Can you work these out from the model? Positions are in its coordinate system, mm. A direction names the side the tool comes from. Coordinates: 2 decimals unless noted, no trailing zeros. Order: outer loops, then holes, each group sorted by start corner. A loop starts at its lowest first (then second) coordinate and runs counter-clockwise, first axis right, second up. Notation, with made-up numbers: (5.5, 87.25) -> (40.5, 87.25) arc R38 ccw to (40.5, 125.25) -> close; hole circle Ø5 at (5, 67.25). An arc over 180 degrees is marked (long way). Answer in a Markdown table with one row per item. Add a question column.
1. Imagine slicing it at C-C on y = 82.5. Write out the boundary of the cut face in (x, z).
2. We'd pull the mould along Y, two halves only. Please class faces 3 (the face through (-2, 29, 25)), 4 (the face through (71, -82, 13)), 5 (the face through (-2, -122.5, 12)): pulls with the +Y half, pulls with the -Y half, needs draft (parallel to the pull), parting line crosses it, or undercut.
3. Will these pins go through, and if not, where does the flat tip stop? pin 1 (15.5 mm diameter, centred on x = 120, y = 82.5, fed in from -Z); pin 2 (8.5 mm diameter, centred on x = 124, y = 82.5, fed in from +Z).
4. Imagine slicing it at B-B on y = 0. Write out the boundary of the cut face in (x, z), plus the area to 3 significant figures.
5. Imagine slicing it at D-D on x = 65. Write out the boundary of the cut face in (y, z).
6. On a 3-axis mill with a long thin cutter (end or side, diameter ignored), from which of +Z, -Z, +X, -X, +Y, -Y can I reach the whole of each face in a straight line? I mean faces 1 (the face through (-114, 83, 13)), 2 (the face through (-2, 122.5, 12)). Say none if no direction works.
7. Imagine slicing it at A-A on x = 0. Write out the boundary of the cut face in (y, z), plus the area to 4 significant figures.
8. If I drill on line 1 along X through (y, z) = (82.5, 4.75); line 2 along X through (y, z) = (-82.5, 7.5); line 3 along Y through (x, z) = (-65, 4.75), over which ranges is the centre line in solid material (lowest first)? Write a range as [from, to].
from build123d import *

# Parameters (mm, degrees)
SKETCH1_W           = 280
SKETCH1_H           = 245
SKETCH1_R           = 5.25
SKETCH1_R_2         = 6
BOSS_EXTRUDE1_DEPTH = 25
SKETCH2_R           = 8.5
CUT_EXTRUDE1_DEPTH  = 12


with BuildPart() as part:
    # Sketch1 → Boss-Extrude1 (new body)
    with BuildSketch(Plane.XY):
        Rectangle(SKETCH1_W, SKETCH1_H)
        with Locations((-120, 82.5)):
            Circle(SKETCH1_R, mode=Mode.SUBTRACT)
        with Locations((120, 82.5)):
            Circle(SKETCH1_R, mode=Mode.SUBTRACT)
        with Locations((-65, -82.5)):
            Circle(SKETCH1_R, mode=Mode.SUBTRACT)
        with Locations((65, -82.5)):
            Circle(SKETCH1_R, mode=Mode.SUBTRACT)
        Circle(SKETCH1_R_2, mode=Mode.SUBTRACT)
    extrude(amount=BOSS_EXTRUDE1_DEPTH)

    # Sketch2 → Cut-Extrude1 (cut)
    with BuildSketch(Plane.XY.offset(25)):
        with Locations((-120, 82.5)):
            Circle(SKETCH2_R)
        with Locations((120, 82.5)):
            Circle(SKETCH2_R)
        with Locations((65, -82.5)):
            Circle(SKETCH2_R)
        with Locations((-65, -82.5)):
            Circle(SKETCH2_R)
    extrude(amount=-CUT_EXTRUDE1_DEPTH, mode=Mode.SUBTRACT)


solid = part.part
Answers follow:
| question | item | result |
|---|---|---|
| 1 | outline | (-140, 0) -> (-125.25, 0) -> (-125.25, 13) -> (-128.5, 13) -> (-128.5, 25) -> (-140, 25) -> close; (-114.75, 0) -> (114.75, 0) -> (114.75, 13) -> (111.5, 13) -> (111.5, 25) -> (-111.5, 25) -> (-111.5, 13) -> (-114.75, 13) -> close; (125.25, 0) -> (140, 0) -> (140, 25) -> (128.5, 25) -> (128.5, 13) -> (125.25, 13) -> close |
| 2 | face 3 | needs draft |
| 2 | face 4 | undercut |
| 2 | face 5 | pulls with the -Y half |
| 3 | pin 1 | stops at z = 0 |
| 3 | pin 2 | stops at z = 13 |
| 4 | outline | (-140, 0) -> (-6, 0) -> (-6, 25) -> (-140, 25) -> close; (6, 0) -> (140, 0) -> (140, 25) -> (6, 25) -> close |
| 4 | area | 6,700 mm² |
| 5 | outline | (-122.5, 0) -> (-87.75, 0) -> (-87.75, 13) -> (-91, 13) -> (-91, 25) -> (-122.5, 25) -> close; (-77.25, 0) -> (122.5, 0) -> (122.5, 25) -> (-74, 25) -> (-74, 13) -> (-77.25, 13) -> close |
| 6 | face 1 | +Z |
| 6 | face 2 | +Z, -Z, +X, -X, +Y |
| 7 | outline | (-122.5, 0) -> (-6, 0) -> (-6, 25) -> (-122.5, 25) -> close; (6, 0) -> (122.5, 0) -> (122.5, 25) -> (6, 25) -> close |
| 7 | area | 5,825 mm² |
| 8 | line 1 | x = [-140, -125.25], [-114.75, 114.75], [125.25, 140] |
| 8 | line 2 | x = [-140, -70.25], [-59.75, 59.75], [70.25, 140] |
| 8 | line 3 | y = [-122.5, -87.75], [-77.25, 122.5] |
